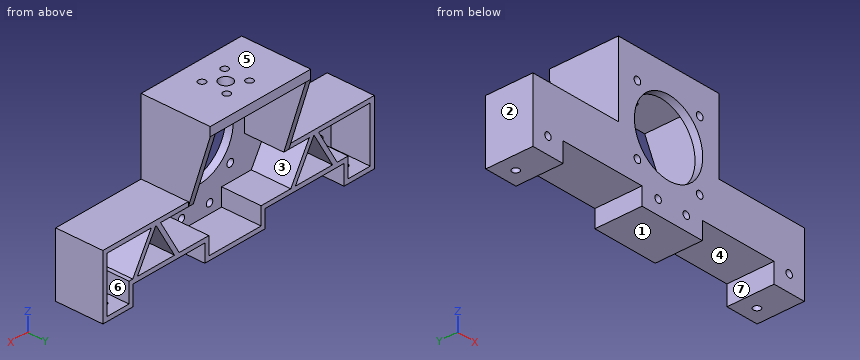
```python
from build123d import *

# Parameters (mm, degrees)
SKETCH_2_R          = 1.6
SKETCH_2_R_2        = 17
SKETCH_2_R_3        = 1.65
EXTRUDE_2_DEPTH     = 3.5
EXTRUDE_3_DEPTH     = 18
EXTRUDE_4_DEPTH     = 10
CUT_EXTRUDE_5_DEPTH = 117.156532317
SKETCH_10_R         = 3
SKETCH_10_R_2       = 1.65
CUT_EXTRUDE_4_DEPTH = 5
EXTRUDE_5_DEPTH     = 18
SKETCH_14_R         = 1.65
CUT_EXTRUDE_6_DEPTH = 10


with BuildPart() as part:
    # 草图2 → 凸台-拉伸2 (new body)
    with BuildSketch(Plane(origin=(0, 0, 0), x_dir=(1, 0, 0), z_dir=(0, 1, 0))):
        Polygon((-42.5, 33.8), (-42.5, 62.8), (-27.5, 62.8), (-27.5, 53.8), (11.8, 53.8), (11.8, 61.8), (41.8, 61.8), (41.8, 53.8), (77.5, 53.8), (77.5, 62.8), (92.5, 62.8), (92.5, 33.8), (50, 33.8), (50, 0), (0, 0), (0, 33.8), align=None)
        with Locations(Location((-35, 55.365042575, 0), (0, 0, 270))):
            Circle(SKETCH_2_R, mode=Mode.SUBTRACT)
        with Locations(Location((85, 55.365042575, 0), (0, 0, 270))):
            Circle(SKETCH_2_R, mode=Mode.SUBTRACT)
        with Locations(Location((19.8, 55.365042575, 0), (0, 0, 270))):
            Circle(SKETCH_2_R, mode=Mode.SUBTRACT)
        with Locations(Location((33.8, 55.365042575, 0), (0, 0, 270))):
            Circle(SKETCH_2_R, mode=Mode.SUBTRACT)
        with Locations(Location((25, 28.8, 0), (0, 0, 270))):
            Circle(SKETCH_2_R_2, mode=Mode.SUBTRACT)
        with Locations(Location((40.5, 44.3, 0), (0, 0, 270))):
            Circle(SKETCH_2_R_3, mode=Mode.SUBTRACT)
        with Locations(Location((40.5, 13.3, 0), (0, 0, 270))):
            Circle(SKETCH_2_R_3, mode=Mode.SUBTRACT)
        with Locations(Location((9.5, 13.3, 0), (0, 0, 270))):
            Circle(SKETCH_2_R_3, mode=Mode.SUBTRACT)
        with Locations(Location((9.5, 44.3, 0), (0, 0, 270))):
            Circle(SKETCH_2_R_3, mode=Mode.SUBTRACT)
    extrude(amount=EXTRUDE_2_DEPTH)

    # 草图6 → 凸台-拉伸3 (add)
    with BuildSketch(Plane(origin=(0, 3.5, 0), x_dir=(1, 0, 0), z_dir=(0, 1, 0))):
        Polygon((11.8, 53.8), (-27.5, 53.8), (-27.5, 62.8), (-42.5, 62.8), (-42.5, 33.8), (0, 33.8), (0, 0), (50, 0), (50, 33.8), (92.5, 33.8), (92.5, 62.8), (77.5, 62.8), (77.5, 53.8), (41.8, 53.8), (41.8, 61.8), (11.8, 61.8), align=None)
        Polygon((13.8, 51.8), (-29.5, 51.8), (-29.5, 60.8), (-40.5, 60.8), (-40.5, 35.8), (2.5, 35.8), (2.5, 4), (47.5, 4), (47.5, 35.8), (90.5, 35.8), (90.5, 60.8), (79.5, 60.8), (79.5, 51.8), (39.8, 51.8), (39.8, 59.8), (13.8, 59.8), align=None, mode=Mode.SUBTRACT)
    extrude(amount=EXTRUDE_3_DEPTH)

    # 草图11 → 凸台-拉伸4 (add)
    with BuildSketch(Plane(origin=(0, 21.5, 0), x_dir=(1, 0, 0), z_dir=(0, 1, 0))):
        Polygon((2.5, 35.8), (2.5, 4), (47.5, 4), (47.5, 35.8), (50, 35.8), (50, 0), (0, 0), (0, 35.8), align=None)
    extrude(amount=EXTRUDE_4_DEPTH)

    # 草图12 → 切除-拉伸5 (cut, through all)
    with BuildSketch(Plane.ZY):
        Polygon((-35.8, 21.5), (-4, 31.5), (-35.8, 31.5), align=None)
    extrude(amount=-CUT_EXTRUDE_5_DEPTH, mode=Mode.SUBTRACT)

    # 草图10 → 切除-拉伸4 (cut)
    with BuildSketch(Plane.XY):
        with Locations((25, 15.656854249)):
            Circle(SKETCH_10_R)
        with Locations((30.656854249, 21.313708499)):
            Circle(SKETCH_10_R_2)
        with Locations((30.656854249, 10)):
            Circle(SKETCH_10_R_2)
        with Locations((19.343145751, 10)):
            Circle(SKETCH_10_R_2)
        with Locations((19.343145751, 21.313708499)):
            Circle(SKETCH_10_R_2)
    extrude(amount=-CUT_EXTRUDE_4_DEPTH, mode=Mode.SUBTRACT)

    # 草图13 → 凸台-拉伸5 (add)
    with BuildSketch(Plane(origin=(0, 3.5, 0), x_dir=(1, 0, 0), z_dir=(0, 1, 0))):
        Polygon((-12.5, 35.8), (-21.737604307, 51.8), (-24.047005384, 51.8), (-14.809401077, 35.8), align=None)
        Polygon((-3.262395693, 51.8), (-12.5, 35.8), (-10.190598923, 35.8), (-0.952994616, 51.8), align=None)
        Polygon((54.552994616, 51.8), (63.790598923, 35.8), (66.1, 35.8), (56.862395693, 51.8), align=None)
        Polygon((75.337604307, 51.8), (66.1, 35.8), (68.409401077, 35.8), (77.647005384, 51.8), align=None)
    extrude(amount=EXTRUDE_5_DEPTH)

    # 草图14 → 切除-拉伸6 (cut)
    with BuildSketch(Plane(origin=(0, 0, -62.8), x_dir=(-1, 0, 0), z_dir=(0, 0, -1))):
        with Locations((35, 14.7)):
            Circle(SKETCH_14_R)
        with Locations(Location((-85, 14.7, 0), (0, 0, 180))):
            Circle(SKETCH_14_R)
    extrude(amount=-CUT_EXTRUDE_6_DEPTH, mode=Mode.SUBTRACT)


solid = part.part
```
Build history of the part. All positions in model axes, mm. Face numbers are marked on the shaded views. A direction names the side the tool comes from. Coordinates: 2 decimals unless noted, no trailing zeros. Write each loop counter-clockwise with the first axis right and the second up, starting at its lowest first coordinate (ties: lowest second). Pieces come first, ordered by that corner, then holes.
1. Band-saw the part on B-B, the plane x = 25. Give the cut face in (y, z).
Answer block:
outline: (0, -61.8) - (21.5, -61.8) - (21.5, -59.8) - (3.5, -59.8) - (3.5, -45.8) - (0, -45.8) - close; (0, -11.8) - (3.5, -11.8) - (3.5, -4) - (12.66, -4) - (12.66, 0) - (0, 0) - close; (18.66, -4) - (31.5, -4) - (31.5, 0) - (18.66, 0) - close
2. Band-saw the part on A-A, the plane y = 26. Give the cut face in (x, z).
Answer block:
outline: (0, -21.49) - (2.5, -21.49) - (2.5, -4) - (47.5, -4) - (47.5, -21.49) - (50, -21.49) - (50, 0) - (0, 0) - close
3. Pull direction Z, two halves, no side cores. Call the marked faces 4, 5, 6 and 7: released by +Z, released by -Z, zero draft, split by the parting line, or undercut.
Answer block:
face 4: released by -Z
face 5: released by +Z
face 6: undercut
face 7: zero draft
4. Drop flat-ended pins along their axis: pin 1 (6 mm diameter, centred on x = -12, y = 16, fed in from +Z); pin 2 (11 mm diameter, centred on x = 80.5, z = -49, fed in from +Y); pin 3 (14 mm diameter, centred on y = 19, z = -24, fed in from -X). Give the stop position or say it passes through.
Answer block:
pin 1: stops at z = -33.8
pin 2: stops at y = 21.5
pin 3: stops at x = 0
5. Drill centre lines: probe 1 along X at (y, z) = (28, -7); probe 2 along X at (y, z) = (11, -39); probe 3 along X at (y, z) = (12.5, -53). Where is each one in solid material? Low to high.
Answer block:
probe 1: x = 0 to 2.5, 47.5 to 50
probe 2: x = -42.5 to -40.5, -16.66 to -14.35, -10.65 to -8.34, 61.94 to 64.25, 67.95 to 70.26, 90.5 to 92.5
probe 3: x = -42.5 to -40.5, -29.5 to 13.8, 39.8 to 79.5, 90.5 to 92.5
6. 3-axis set-ups, long thin cutter, end or side, ignore diameter. For the marked faces 1, 2 and 3: which of +Z, -Z, +X, -X, +Y, -Y reach the whole face in a straight line?
Answer block:
face 1: -Z, +Y, -Y
face 2: +Z, -Z, -X, +Y, -Y
face 3: +Y
7. Band-saw the part on D-D, the plane x = 52. Give the cut face in (y, z), and give its area (3 significant figures).
Answer block:
outline: (0, -53.8) - (21.5, -53.8) - (21.5, -51.8) - (3.5, -51.8) - (3.5, -35.8) - (21.5, -35.8) - (21.5, -33.8) - (0, -33.8) - close
area: 142 mm2
8. Band-saw the part on C-C, the plane z = -41. Give the cut face in (x, y), and give its area (3 significant figures).
Answer block:
outline: (-42.5, 0) - (13.16, 0) - (13.16, 3.5) - (-7.19, 3.5) - (-7.19, 21.5) - (-9.5, 21.5) - (-9.5, 3.5) - (-15.5, 3.5) - (-15.5, 21.5) - (-17.81, 21.5) - (-17.81, 3.5) - (-40.5, 3.5) - (-40.5, 21.5) - (-42.5, 21.5) - close; (36.84, 0) - (92.5, 0) - (92.5, 21.5) - (90.5, 21.5) - (90.5, 3.5) - (71.41, 3.5) - (71.41, 21.5) - (69.1, 21.5) - (69.1, 3.5) - (63.1, 3.5) - (63.1, 21.5) - (60.79, 21.5) - (60.79, 3.5) - (36.84, 3.5) - close
area: 628 mm2
